Verification items for this drawing (mm, ordinates from the low corner). A direction names the side the tool comes from. Give positions to 0.01 mm unless a question says otherwise; leave off trailing zeros. Order: outer loops, then holes, each group sorted by start corner. A loop starts at its lowest first (then second) coordinate and runs counter-clockwise, first axis right, second up. Notation, with made-up numbers: M 85.25,64 L 141.25,64 A38 ccw 141.25,102 Z; hole C -33,-8 d10. An arc over 180 degrees is marked long. Return JSON: item names as keys, results as strings. Group by question number.
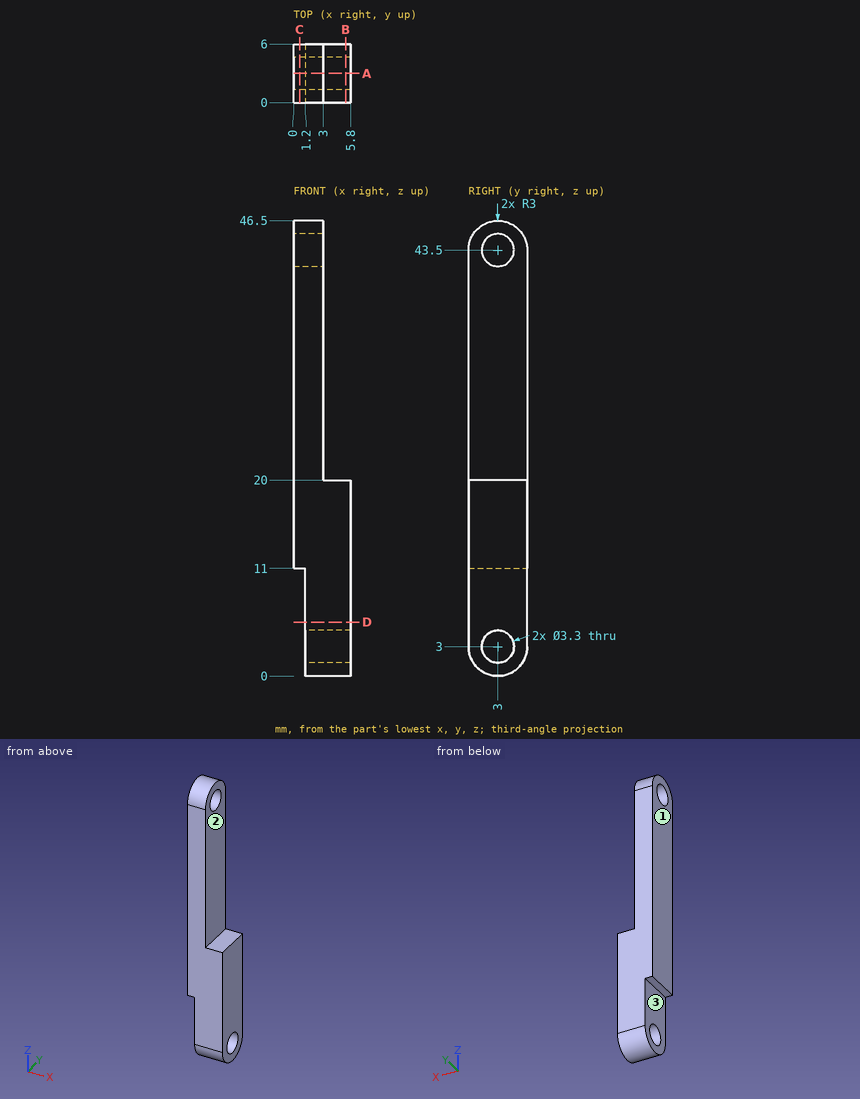
1) Depth check by flat-ended pin: P1, Ø2.5, axis at y = 3, z = 3, coming from the +X side; P2, Ø1, axis at y = 0.5, z = 33, coming from the +X side; P3, Ø1.4, axis at x = 4, y = 2, coming from the +Z side. Enter the tip coordinate at first touch or a pass-through.
2) Sectioned sample at B-B on x = 5.3. Record the boundary of the cut face in (y, z).
3) Sectioned sample at A-A on y = 3. Record the boundary of the cut face in (x, z).
4) Material ranges on line 1 along Y through (x, z) = (1.55, 43.5); line 2 along Z through (x, y) = (3.6, 3); line 3 along X through (y, z) = (5.6, 5.5), recorded low to high.
5) Tool access check on the marked faces 1, 2 and 3. Record the directions out of +Z, -Z, +X, -X, +Y, -Y that give a thin tool (end or side, any length) a straight path to the whole face; none if there is none.
6) Sectioned sample at D-D on z = 5.5. Record the boundary of the cut face in (x, y).
7) Sectioned sample at C-C on x = 0.6. Record the boundary of the cut face in (y, z), then the cut area to 3 significant figures.
Reply:
{
 "1": {"P1": "through", "P2": "x = 3", "P3": "z = 20"},
 "2": {"outline": "M 0,3 A3 ccw 6,3 L 6,20 L 0,20 Z; hole C 3,3 d3.3"},
 "3": {"outline": "M 0,11 L 1.2,11 L 1.2,4.65 L 5.8,4.65 L 5.8,20 L 3,20 L 3,41.85 L 0,41.85 Z; M 0,45.15 L 3,45.15 L 3,46.5 L 0,46.5 Z; M 1.2,0 L 5.8,0 L 5.8,1.35 L 1.2,1.35 Z"},
 "4": {"line 1": "0 to 1.35, 4.65 to 6", "line 2": "0 to 1.35, 4.65 to 20", "line 3": "1.2 to 5.8"},
 "5": {"face 1": "+Z, -Z, -X, +Y, -Y", "face 2": "+Z, +X, +Y, -Y", "face 3": "-Z, -X, +Y, -Y"},
 "6": {"outline": "M 1.2,0 L 5.8,0 L 5.8,6 L 1.2,6 Z"},
 "7": {"outline": "M 0,11 L 6,11 L 6,43.5 A3 ccw 0,43.5 Z; hole C 3,43.5 d3.3", "area": "201 mm^2"}
}
